Source: CAD feature listing. Evaluate the final solid. Frame: model axes, mm. Face numbers are marked on the shaded views. A direction names the side the tool comes from. Coordinates: 2 decimals unless noted, no trailing zeros. Write each loop counter-clockwise with the first axis right and the second up, starting at its lowest first coordinate (ties: lowest second). Pieces come first, ordered by that corner, then holes. Notation, with made-up numbers: (34, 80.25) - (42, 80.25) arc R16 ccw to (42, 107.25) - close; hole circle Ø1 at (-23.5, 55). An arc over 180 degrees is marked (long way). One line per item, written item: value.
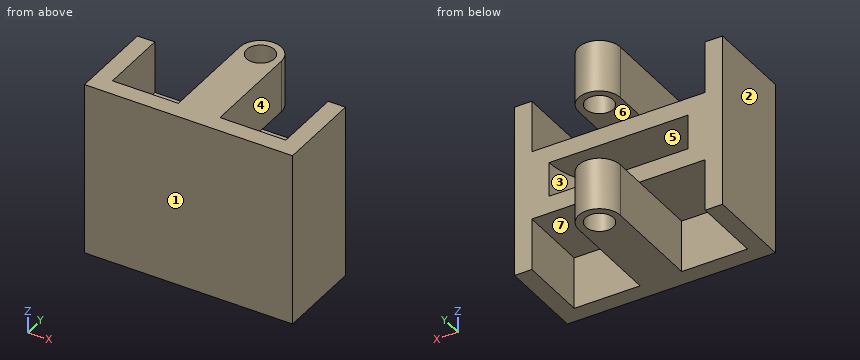
Autodesk Inventor part; units mm, degrees
ref_plane "Work Plane1" through (0, 0, 25) normal (0, 0, 1) x (1, 0, 0)
ref_plane "YZ Plane" through (0, 0, 0) normal (1, 0, 0) x (0, 1, 0)
ref_plane "XZ Plane" through (0, 0, 0) normal (0, 1, 0) x (-1, 0, 0)
sketch "Sketch2" plane through (0, 0, 0) normal (0, 0, 1) x (1, 0, 0)
  line L0 (30, -13.3137) -> (-30, -13.3137)
  line L1 (-30, -13.3137) -> (-30, 11.6863)
  line L2 (30, 11.6863) -> (30, -13.3137)
  line L3 (-25, 11.6863) -> (-30, 11.6863)
  line L4 (-6, 11.6863) -> (-6, 20.6863)
  line L5 (6, 20.6863) -> (6, 11.6863)
  arc A0 (6, 20.6863) -> (-6, 20.6863) centre (0, 20.6863) ccw
  circle A1 centre (0, 20.6863) radius 4
  line L6 (-30, 11.6863) -> (-6, 11.6863)
  line L7 (6, 11.6863) -> (30, 11.6863)
  point P0 (0, 0)
  dimension "d0" = 60
  dimension "d9" = 25
  dimension "d12" = 8
  dimension "d13" = 12
  dimension "d14" = 9
extrude "Extrusion1" add sketch "Sketch2" along normal blind 25
sketch "Sketch3" plane through (0, 0, 0) normal (0, 0, -1) x (-1, 0, 0)
  line L0 (-25, 11.6863) -> (-6, 11.6863)
  line L1 (-6, 11.6863) -> (-6, -8.3137)
  line L2 (-6, -8.3137) -> (-25, -8.3137)
  line L3 (-25, -8.3137) -> (-25, 11.6863)
  line L4 (25, 11.6863) -> (6, 11.6863)
  line L5 (6, 11.6863) -> (6, -8.3137)
  line L6 (6, -8.3137) -> (25, -8.3137)
  line L7 (25, -8.3137) -> (25, 11.6863)
  line L8 (30, -13.3137) -> (-30, -13.3137)
  line L9 (-30, -13.3137) -> (-30, 11.6863)
  line L10 (30, 11.6863) -> (30, -13.3137)
  point P0 (0, 0)
  point P1 (-30, -0.8137)
  dimension "d17" = 5
  dimension "d18" = 5
  dimension "d19" = 5
  dimension "d20" = 5
extrude "Extrusion2" cut sketch "Sketch3" against normal blind 15
sketch "Sketch4" plane through (0, 0, 25) normal (0, 0, 1) x (1, 0, 0)
  line L0 (-6, 11.6863) -> (6, 11.6863)
  line L1 (6, 11.6863) -> (6, 20.6863)
  line L2 (6, 26.6863) -> (0, 26.6863)
  line L3 (-6, 20.6863) -> (-6, 11.6863)
  arc A0 (6, 20.6863) -> (-6, 20.6863) centre (0, 20.6863) ccw
  circle A1 centre (0, 20.6863) radius 4
  point P0 (0, 0)
  dimension "d23" = 15
extrude "Extrusion3" cut sketch "Sketch4" against normal blind 10
sketch "Sketch5" plane through (-30, 11.6863, 25) normal (0, 1, 0) x (1, 0, 0)
  line L0 (0, 0) -> (60, 0)
  line L1 (30, 0) -> (50, 0)
  line L2 (50, 0) -> (50, 5)
  line L3 (50, 5) -> (30, 5)
  line L4 (30, 5) -> (30, 0)
  point P0 (30, 25)
  dimension "d27" = 20
  dimension "d28" = 5
revolve "Revolution1" cut sketch "Sketch5" angle 360 about axis through (0, 11.6863, 20) along (0, 0, 1)
ref_plane "Work Plane1" through (0, 0, 25) normal (0, 0, 1) x (1, 0, 0)
mirror "Mirror1" about plane through (0, 0, 25) normal (0, 0, 1)
properties part number "khurramf_01_Base"
1) Section query D-D on x = -8.5. Output: boundary loops of the cut face in (y, z).
Values found:
outline: (-13.31, 0) - (-8.31, 0) - (-8.31, 15) - (11.69, 15) - (11.69, 20) - (-6.42, 20) - (-6.42, 30) - (11.69, 30) - (11.69, 35) - (-8.31, 35) - (-8.31, 50) - (-13.31, 50) - close
2) Reachability of the marked faces 4, 5, 6 and 7 from +Z, -Z, +X, -X, +Y, -Y: full face, straight path, thin tool, end or side. Return the list, or none.
Values found:
face 4: +Z, +Y
face 5: +Y
face 6: +X, -X, +Y
face 7: -Z, +Y
3) Contact query for flat-ended pins moving along their axis: P1, Ø6, axis at x = -2, y = 22.5, coming from the +Z side; P2, Ø4, axis at x = 11, y = -5.5, coming from the +Z side; P3, Ø6, axis at y = 15, z = 10.5, coming from the -X side; P4, Ø7.5, axis at x = -12.5, z = 8.5, coming from the +Y side. Output: stop coordinate, or through.
Values found:
P1: z = 50
P2: z = 35
P3: x = -6
P4: y = -8.31
4) Section query A-A on x = 0. Output: boundary loops of the cut face in (y, z), then the cut area to 3 significant figures.
Values found:
outline: (-13.31, 0) - (16.69, 0) - (16.69, 15) - (11.69, 15) - (11.69, 20) - (-8.31, 20) - (-8.31, 30) - (11.69, 30) - (11.69, 35) - (16.69, 35) - (16.69, 50) - (-13.31, 50) - close; (24.69, 0) - (26.69, 0) - (26.69, 15) - (24.69, 15) - close; (24.69, 35) - (26.69, 35) - (26.69, 50) - (24.69, 50) - close
area: 1,260 mm2
5) Section query C-C on y = 1. Output: boundary loops of the cut face in (x, z), then the cut area to 3 significant figures.
Values found:
outline: (-30, 0) - (-25, 0) - (-25, 15) - (-6, 15) - (-6, 0) - (6, 0) - (6, 15) - (25, 15) - (25, 0) - (30, 0) - (30, 50) - (25, 50) - (25, 35) - (6, 35) - (6, 50) - (-6, 50) - (-6, 35) - (-25, 35) - (-25, 50) - (-30, 50) - close; hole (-16.91, 20) - (16.91, 20) - (16.91, 30) - (-16.91, 30) - close
area: 1,520 mm2
6) Material intervals for line 1 (X direction, y = -6, z = 40); line 2 (Y direction, x = 0, z = 42); line 3 (Z direction, x = -6.5, y = 10), sorted ascending.
Values found:
line 1: -30 to -25, -6 to 6, 25 to 30
line 2: -13.31 to 16.69, 24.69 to 26.69
line 3: 15 to 20, 30 to 35
7) Draft query along X for the marked faces 1, 2 and 3. Return one class per face: released by +X, released by -X, zero draft, split by the parting line, or undercut.
Values found:
face 1: zero draft
face 2: released by -X
face 3: undercut
8) Section query B-B on z = 13.5. Output: boundary loops of the cut face in (x, y).
Values found:
outline: (-30, -13.31) - (30, -13.31) - (30, 11.69) - (25, 11.69) - (25, -8.31) - (6, -8.31) - (6, 20.69) arc R6 ccw to (-6, 20.69) - (-6, -8.31) - (-25, -8.31) - (-25, 11.69) - (-30, 11.69) - close; hole circle Ø8 at (0, 20.69)
